Geometry: see drawing. Coordinates: mm, zero at the bounding-box minimum. Coordinates: 2 decimals unless noted, no trailing zeros. Loops run counter-clockwise (first coordinate to the right, second up) from the corner with the lowest first, then second, coordinate; pieces in that order, holes last. Notation, with made-up numbers: M 44.25,-40 L 85.25,-40 A19 cw 85.25,-15 Z; hole C 44,87 d9. An arc over 180 degrees is marked long. One line per question, with ' | ' between items. Start each with the question number.
1. Section query A-A, the plane y = 1.35. Output: boundary loops of the cut face in (x, z).
2. Ray query, probe 1 along X at (y, z) = (1.7, 13); probe 2 along X at (y, z) = (2.1, 91.5); probe 3 along X at (y, z) = (1.45, 82). Return the intervals inside material, ascending.
3. Pin query (flat end, axial travel): P1, Ø6, axis at x = 150, z = 13, coming from the -Y side; P2, Ø4.5, axis at x = 20, z = 107, coming from the -Y side. Return the tip coordinate at first contact, or that it passes through.
4. Section query B-B, the plane z = 13. Output: boundary loops of the cut face in (x, y), and give its area (3 significant figures).
5. Section query C-C, the plane x = 20. Output: boundary loops of the cut face in (y, z), and give its area (3 significant figures).
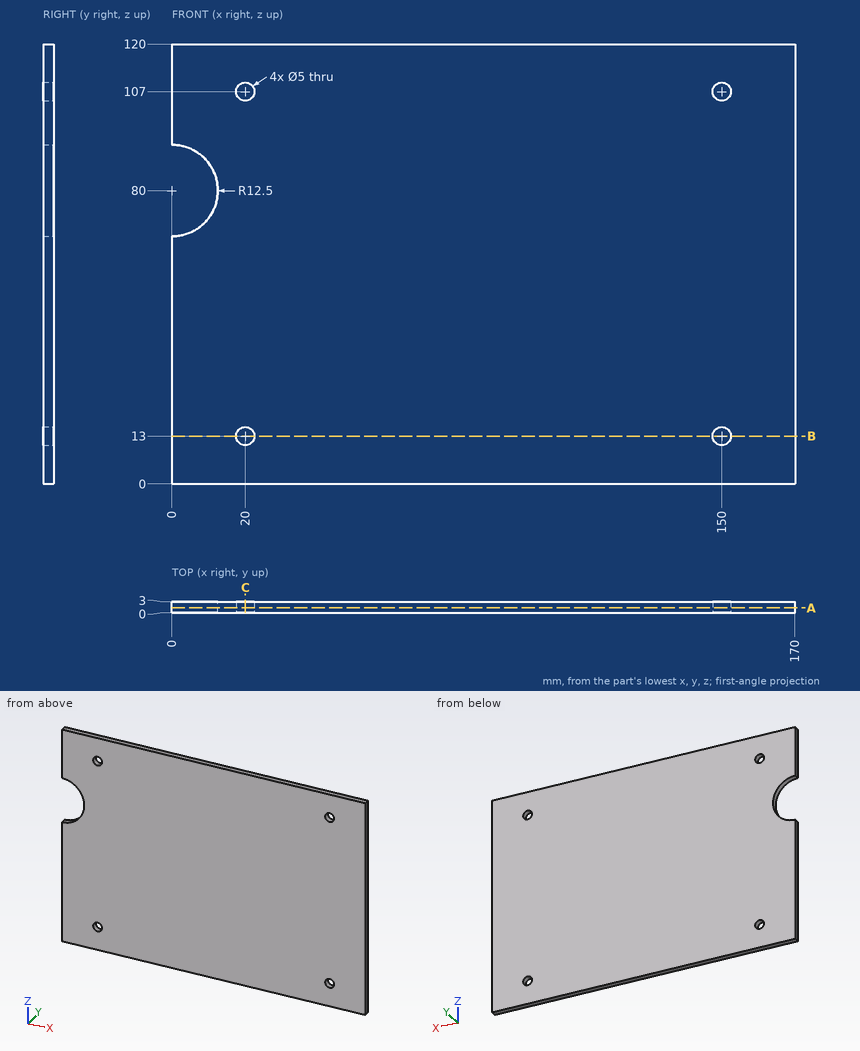
Taken from the geometry:
1) outline: M 0,0 L 170,0 L 170,120 L 0,120 L 0,92.5 A12.5 cw 0,67.5 Z; hole C 20,13 d5; hole C 20,107 d5; hole C 150,13 d5; hole C 150,107 d5
2) probe 1: 0 to 17.5, 22.5 to 147.5, 152.5 to 170 | probe 2: 4.9 to 170 | probe 3: 12.34 to 170
3) P1: y = 0 | P2: through
4) outline: M 0,0 L 17.5,0 L 17.5,3 L 0,3 Z; M 22.5,0 L 147.5,0 L 147.5,3 L 22.5,3 Z; M 152.5,0 L 170,0 L 170,3 L 152.5,3 Z | area: 480 mm^2
5) outline: M 0,0 L 3,0 L 3,10.5 L 0,10.5 Z; M 0,15.5 L 3,15.5 L 3,104.5 L 0,104.5 Z; M 0,109.5 L 3,109.5 L 3,120 L 0,120 Z | area: 330 mm^2
